Here's how the part is built. I have some questions about the finished solid (model axes, mm). A direction names the side the tool comes from. Give positions to 0.01 mm unless a question says otherwise; leave off trailing zeros. Loops run counter-clockwise (first coordinate to the right, second up) from the corner with the lowest first, then second, coordinate; pieces in that order, holes last. Notation, with made-up numbers: M 24,83 L 60,83 A14 cw 60,99 Z; hole C 75,57 d10. An arc over 180 degrees is marked long. Answer as CSV lines item,"result". Start each with the question number.
Item 1: If I drill on line 1 along Z through (x, y) = (29, -51); line 2 along Z through (x, y) = (29, -55.25); line 3 along Y through (x, z) = (22, -103.5), over which ranges is the centre line in solid material (lowest first)? Write a range as from..to.
Item 2: For faces 1 (the flat face through (22, -40.5, 14)), 2 (the cylindrical face through (29.406, -56.604, 35.534)), 3 (the flat face through (22, -40.5, -104)), which set-ups out of +Z, -Z, +X, -X, +Y, -Y let a thin tool reach every point of the face, with its end or its side?
Item 3: I want a section at C-C on x = 50. List the corners of the cut face in (y, z) for me, plus the area to 3 significant figures.
Item 4: Will these pins go through, and if not, where does the flat tip stop? P1, Ø10.5, axis at x = 19, z = -102, coming from the +Y side; P2, Ø12, axis at y = -33, z = -93, coming from the +X side; P3, Ø6, axis at x = 42.5, y = -10, coming from the -Z side; P4, Ø1, axis at x = 30.5, z = 20.5, coming from the +Y side.
Item 5: I want a section at A-A on x = 29. List the corners of the cut face in (y, z) for me.
Item 6: If we mould it in two halves opening along Z, with no side actions, what happens to faces 4 (the cylindrical face through (29.406, 42.986, -2.026)), 5 (the flat face through (0, -22, -36)), 6 (the cylindrical face through (29.41, -56.74, -120.94)), 7 (the conical face through (25.46, -44.18, 16.19))? For each: released by +Z, released by -Z, zero draft, split by the parting line, or undercut.
Item 7: I want a section at B-B on z = -4.5. List the corners of the cut face in (x, y) for me, plus the area to 3 significant figures.
Item 8: I want a section at D-D on y = 43. List the corners of the cut face in (x, z) for me, plus the area to 3 significant figures.
from build123d import *

# Parameters (mm, degrees)
F1_DEPTH       = 58
F2_R           = 9
F4_D           = 6.7564
F4_DEPTH       = 127
F4_CSINK_D     = 13.4874
F4_CSINK_ANGLE = 82
F4_TIP         = 2.0298273432


# Not quite as in the source:
# - a feature names something its author has since deleted; it is built from what else it names


with BuildPart() as f1:
    # F0 (on Right) → F1 (new body)
    with BuildSketch(Plane.YZ):
        with BuildLine():
            Line((59.3103850067, 0), (40.5, 0))
            ThreePointArc((40.5, 0), (28.6378246381, -28.6378246381), (0, -40.5))
            ThreePointArc((0, -40.5), (-28.6378246381, -28.6378246381), (-40.5, 0))
            Line((-40.5, 0), (-40.5, -43.3298023263))
            ThreePointArc((-40.5, -43.3298023263), (-23.1030418264, -54.62573778), (-2.8803521713, -59.2404029443))
            ThreePointArc((-2.8803521713, -59.2404029443), (-1.4395179453, -59.2483059491), (0, -59.3103850067))
            ThreePointArc((0, -59.3103850067), (41.938775433, -41.938775433), (59.3103850067, 0))
        make_face()
        with BuildLine():
            Line((-40.5, -43.3298023263), (-40.5, 0))
            Line((-40.5, 0), (-59.3103850067, 0))
            ThreePointArc((-59.3103850067, 0), (-54.4049279129, -23.6183316184), (-40.5, -43.3298023263))
        make_face()
        with BuildLine():
            Line((-59.3103850067, 0), (-40.5, 0))
            Line((-40.5, 0), (-40.5, 38.1))
            Line((-40.5, 38.1), (-45.4545021933, 38.1))
            ThreePointArc((-45.4545021933, 38.1), (-55.7388813801, 20.2706406444), (-59.3103850067, 0))
        make_face()
        with BuildLine():
            Line((-59.3103850067, 38.1), (-59.3103850067, 0))
            ThreePointArc((-59.3103850067, 0), (-55.7388813801, 20.2706406444), (-45.4545021933, 38.1))
            Line((-45.4545021933, 38.1), (-59.3103850067, 38.1))
        make_face()
        with BuildLine():
            ThreePointArc((-40.5, -43.3298023263), (-54.4049279129, -23.6183316184), (-59.3103850067, 0))
            Line((-59.3103850067, 0), (-59.3103850067, -123.6414313316))
            Line((-59.3103850067, -123.6414313316), (-40.5, -123.6414313316))
            Line((-40.5, -123.6414313316), (-40.5, -93.8428338624))
            Line((-40.5, -93.8428338624), (-40.5, -43.3298023263))
        make_face()
        with BuildLine():
            ThreePointArc((-2.8803521713, -59.2404029443), (-23.1030418264, -54.62573778), (-40.5, -43.3298023263))
            Line((-40.5, -43.3298023263), (-40.5, -93.8428338624))
            ThreePointArc((-40.5, -93.8428338624), (-28.3045630471, -69.3504788941), (-2.8803521713, -59.2404029443))
        make_face()
    extrude(amount=F1_DEPTH)

    # F2
    f2_edges = [f1.edges().sort_by_distance(p)[0] for p in [
        (29, -40.5, 38.1),
        (29, -59.310385, 38.1),
        (29, 59.310385, 0),
        (29, 40.5, 0),
        (29, -40.5, -123.641431),
        (29, -59.310385, -123.641431),
    ]]
    fillet(f2_edges, radius=F2_R)

    # F4
    with Locations(Plane(origin=(0, -40.5, 0), x_dir=(-1, 0, 0), z_dir=(0, 1, 0))):
        with Locations((-29, 16.0360112786), (-29, -104.242132597)):
            CounterSinkHole(F4_D / 2, F4_CSINK_D / 2, depth=F4_DEPTH, counter_sink_angle=F4_CSINK_ANGLE)
            with Locations((0, 0, -(F4_DEPTH + F4_TIP / 2))):  # 118° drill point
                Cone(0, F4_D / 2, F4_TIP, mode=Mode.SUBTRACT)


solid = f1.part
Result:
1,line 1,"-123.61..-107.62, -100.86..12.66, 19.41..38.07"
1,line 2,"-122.16..-107.62, -100.86..12.66, 19.41..36.62"
1,line 3,"-59.31..-40.5"
2,face 1,"+Z, +X, -X, +Y"
2,face 2,"+Z, +X, -X, -Y"
2,face 3,"-Z, +X, -X, +Y"
3,outline,"M -59.31,-114.64 A9 ccw -50.31,-123.64 L -49.5,-123.64 A9 ccw -40.5,-114.64 L -40.5,-93.84 A38.31 cw 0,-59.31 A59.31 ccw 58.35,-10.61 A9 ccw 49.5,0 L 48.67,0 A9 ccw 39.82,-7.36 A40.5 cw -40.5,0 L -40.5,29.1 A9 ccw -49.5,38.1 L -50.31,38.1 A9 ccw -59.31,29.1 Z"
3,area,"5,830 mm^2"
4,P1,"y = -40.5"
4,P2,"through"
4,P3,"z = -60.74"
4,P4,"y = -42.27"
5,outline,"M -59.31,-114.64 A9 ccw -50.31,-123.64 L -49.5,-123.64 A9 ccw -40.5,-114.64 L -40.5,-110.99 L -44.37,-107.62 L -59.31,-107.62 Z; M -59.31,-100.86 L -44.37,-100.86 L -40.5,-97.5 L -40.5,-93.84 A38.31 cw 0,-59.31 A59.31 ccw 58.35,-10.61 A9 ccw 49.5,0 L 48.67,0 A9 ccw 39.82,-7.36 A40.5 cw -40.5,0 L -40.5,9.29 L -44.37,12.66 L -59.31,12.66 Z; M -59.31,19.41 L -44.37,19.41 L -40.5,22.78 L -40.5,29.1 A9 ccw -49.5,38.1 L -50.31,38.1 A9 ccw -59.31,29.1 Z"
6,face 4,"released by +Z"
6,face 5,"zero draft"
6,face 6,"released by -Z"
6,face 7,"undercut"
7,outline,"M 0,-59.31 L 58,-59.31 L 58,-40.25 L 0,-40.25 Z; M 0,40.88 L 58,40.88 L 58,57.29 L 0,57.29 Z"
7,area,"2,060 mm^2"
8,outline,"M 0,-40.85 L 58,-40.85 L 58,-2.01 L 0,-2.01 Z"
8,area,"2,250 mm^2"
